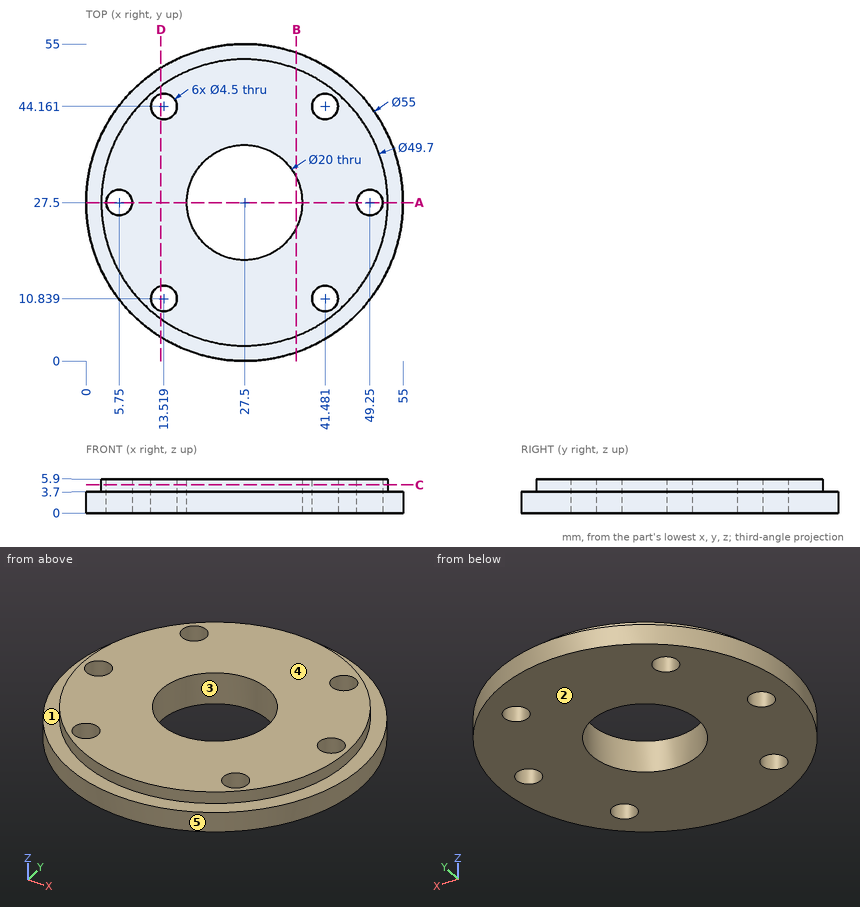
Could you check a few things on this drawing? It's one solid part, dimensions in mm from its lowest x, y, z. A direction names the side the tool comes from. Coordinates: 2 decimals unless noted, no trailing zeros. Write each loop counter-clockwise with the first axis right and the second up, starting at its lowest first coordinate (ties: lowest second). Pieces come first, ordered by that corner, then holes. Notation, with made-up numbers: M 55.5,-40 L 94.5,-40 A6 ccw 94.5,-30 Z; hole C 85.25,-15.75 d6. An arc over 180 degrees is marked long. Answer as CSV lines item,"result". Start each with the question number.
Q1. Suppose I cut it at A-A, the plane y = 27.5. List the corners of the cut face in (x, z) for me, then the cut area to 3 significant figures.
Q2. Suppose I cut it at B-B, the plane x = 36.5. List the corners of the cut face in (y, z) for me (1 decimal).
Q3. I need wall thicknesses on probe 1 along Y at (x, z) = (42.5, 4.75) (1 decimal); probe 2 along X at (y, z) = (28, 0.4) (1 decimal); probe 3 along Y at (x, z) = (35.5, 1.95). Which ranges of each line are inside material? Lowest first, please. Write a range as [from, to].
Q4. If we mould it in two halves opening along Y, with no side actions, what happens to the marked faces 3, 4 and 5? For each: pulls with the +Y half, pulls with the -Y half, needs draft (parallel to the pull), parting line crosses it, or undercut.
Q5. Suppose I cut it at C-C, the plane z = 4.9. List the corners of the cut face in (x, y) for me.
Q6. Will these pins go through, and if not, where does the flat tip stop? pin 1 Ø3 at (y, z) = (43, 4.5) entering from +X; pin 2 Ø3.5 at (x, y) = (13.52, 10.84) entering from -Z; pin 3 Ø1 at (x, z) = (22, 1.5) entering from +Y; pin 4 Ø2 at (y, z) = (19, 3.5) entering from -X.
Q7. Suppose I cut it at D-D, the plane x = 13. List the corners of the cut face in (y, z) for me, then the cut area to 3 significant figures.
Q8. For the marked faces 1 and 2, which set-ups out of +Z, -Z, +X, -X, +Y, -Y let a thin tool reach every point of the face, with its end or its side?
Entries:
1,outline,"M 0,0 L 3.5,0 L 3.5,5.9 L 2.65,5.9 L 2.65,3.7 L 0,3.7 Z; M 8,0 L 17.5,0 L 17.5,5.9 L 8,5.9 Z; M 37.5,0 L 47,0 L 47,5.9 L 37.5,5.9 Z; M 51.5,0 L 55,0 L 55,3.7 L 52.35,3.7 L 52.35,5.9 L 51.5,5.9 Z"
1,area,"142 mm²"
2,outline,"M 1.5,0 L 23.1,0 L 23.1,5.9 L 4.3,5.9 L 4.3,3.7 L 1.5,3.7 Z; M 31.9,0 L 53.5,0 L 53.5,3.7 L 50.7,3.7 L 50.7,5.9 L 31.9,5.9 Z"
3,probe 1,"y = [7.7, 8.8], [12.8, 42.2], [46.2, 47.3]"
3,probe 2,"x = [0, 3.6], [7.9, 17.5], [37.5, 47.1], [51.4, 55]"
3,probe 3,"y = [1.19, 21.5], [33.5, 53.81]"
4,face 3,"undercut"
4,face 4,"needs draft"
4,face 5,"parting line crosses it"
5,outline,"C 27.5,27.5 d49.7; hole C 5.75,27.5 d4.5; hole C 13.52,10.84 d4.5; hole C 13.52,44.16 d4.5; hole C 27.5,27.5 d20; hole C 41.48,10.84 d4.5; hole C 41.48,44.16 d4.5; hole C 49.25,27.5 d4.5"
6,pin 1,"stops at x = 51.03"
6,pin 2,"passes through"
6,pin 3,"stops at y = 54.54"
6,pin 4,"stops at x = 1.04"
7,outline,"M 4.13,0 L 8.65,0 L 8.65,5.9 L 7.32,5.9 L 7.32,3.7 L 4.13,3.7 Z; M 13.03,0 L 41.97,0 L 41.97,5.9 L 13.03,5.9 Z; M 46.35,0 L 50.87,0 L 50.87,3.7 L 47.68,3.7 L 47.68,5.9 L 46.35,5.9 Z"
7,area,"210 mm²"
8,face 1,"+Z"
8,face 2,"-Z, +X, -X, +Y, -Y"
